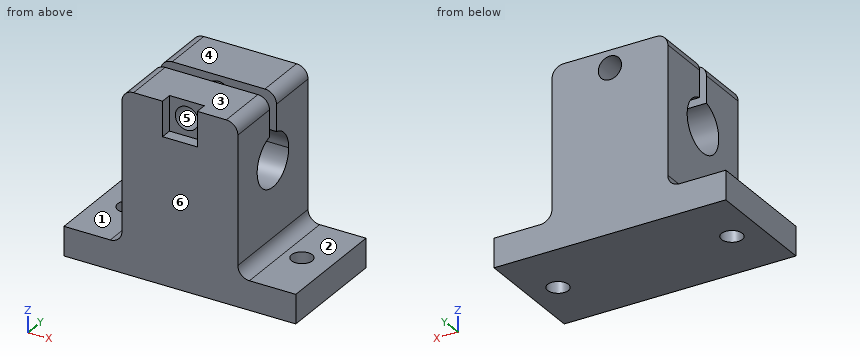
from build123d import *

# Parameters (mm, degrees)
F1_DEPTH = 20
F2_R     = 1.8
F3_DEPTH = 25
F5_DEPTH = 25
F7_DEPTH = 6
F8_R     = 2
F9_DEPTH = 25
F10_R    = 2


with BuildPart() as f1:
    # F0 (on Front) → F1 (new body)
    with BuildSketch(Plane.XZ):
        Polygon((10, 31), (-10, 31), (-10, 5), (-20, 5), (-20, 0), (20, 0), (20, 5), (10, 5), align=None)
    extrude(amount=F1_DEPTH)

    # F2 (on face) → F3 (cut)
    with BuildSketch(Plane(origin=(0, 0, 0), x_dir=(1, 0, 0), z_dir=(0, 0, -1))):
        with Locations((-15, 10)):
            Circle(F2_R)
        with Locations((15, 10)):
            Circle(F2_R)
    extrude(amount=-F3_DEPTH, mode=Mode.SUBTRACT)

    # F4 (on face) → F5 (cut)
    with BuildSketch(Plane.YZ.offset(10)):
        with BuildLine():
            ThreePointArc((-11, 24.3874821937), (-12.8062430401, 16.4821881801), (-5.5, 20))
            ThreePointArc((-5.5, 20), (-6.4821881801, 22.8062430401), (-9, 24.3874821937))
            Line((-9, 24.3874821937), (-9, 20))
            Line((-9, 20), (-10, 20))
            Line((-10, 20), (-11, 20))
            Line((-11, 20), (-11, 24.3874821937))
        make_face()
        with BuildLine():
            ThreePointArc((-11, 24.3874821937), (-10, 24.5), (-9, 24.3874821937))
            Line((-9, 24.3874821937), (-9, 31))
            Line((-9, 31), (-11, 31))
            Line((-11, 31), (-11, 24.3874821937))
        make_face()
        with BuildLine():
            Line((-9, 20), (-9, 24.3874821937))
            ThreePointArc((-9, 24.3874821937), (-10, 24.5), (-11, 24.3874821937))
            Line((-11, 24.3874821937), (-11, 20))
            Line((-11, 20), (-10, 20))
            Line((-10, 20), (-9, 20))
        make_face()
    extrude(amount=-F5_DEPTH, mode=Mode.SUBTRACT)

    # F6 (on face) → F7 (cut)
    with BuildSketch(Plane.XY.offset(31)):
        Polygon((-3, -18), (-3, -20), (3, -20), (3, -18), (0, -18), align=None)
    extrude(amount=-F7_DEPTH, mode=Mode.SUBTRACT)

    # F8 (on face) → F9 (cut)
    with BuildSketch(Plane.XZ.offset(18)):
        with Locations((0, 28)):
            Circle(F8_R)
    extrude(amount=-F9_DEPTH, mode=Mode.SUBTRACT)

    # F10
    f10_edges = [f1.edges().sort_by_distance(p)[0] for p in [
        (10, -15.5, 31),
        (10, -4.5, 31),
        (-10, -4.5, 31),
        (-10, -15.5, 31),
        (10, -10, 5),
        (-10, -10, 5),
    ]]
    fillet(f10_edges, radius=F10_R)


solid = f1.part
Read the model definition and answer for the solid it produces. Units are mm, in the model's axes. Face numbers are marked on the shaded views. A direction names the side the tool comes from. Give positions to 0.01 mm unless a question says otherwise; leave off trailing zeros. Loops run counter-clockwise (first coordinate to the right, second up) from the corner with the lowest first, then second, coordinate; pieces in that order, holes last. Notation, with made-up numbers: M 12,60.25 L 46,60.25 A30 ccw 46,87.25 Z; hole C -25.5,89.5 d10. An arc over 180 degrees is marked long. Write each question's results on one line, items separated by ' | '.
1. Section A-A on y = -10 is taken. Give the vertices of the cut face in (x, z).
Values:
outline: M -20,0 L -16.8,0 L -16.8,5 L -20,5 Z; M -13.2,0 L 13.2,0 L 13.2,5 L 12,5 A2 cw 10,7 L 10,15.5 L -10,15.5 L -10,7 A2 cw -12,5 L -13.2,5 Z; M 16.8,0 L 20,0 L 20,5 L 16.8,5 Z
2. Section B-B on x = 0 is taken. Give the vertices of the cut face in (y, z).
Values:
outline: M -20,0 L 0,0 L 0,26 L -9,26 L -9,24.39 A4.5 cw long -11,24.39 L -11,26 L -18,26 L -18,25 L -20,25 Z; M -18,30 L -11,30 L -11,31 L -18,31 Z; M -9,30 L 0,30 L 0,31 L -9,31 Z
3. Section C-C on y = -15.5 is taken. Give the vertices of the cut face in (x, z), plus the area to 3 significant figures.
Values:
outline: M -20,0 L 20,0 L 20,5 L 12,5 A2 cw 10,7 L 10,29 A2 ccw 8,31 L -8,31 A2 ccw -10,29 L -10,7 A2 cw -12,5 L -20,5 Z; hole C 0,28 d4 | area: 707 mm^2
4. The mould has two halves that part along Z. Classify the marked faces 4, 5 and 6: pulls with the +Z half, pulls with the -Z half, needs draft (parallel to the pull), parting line crosses it, or undercut.
Values:
face 4: pulls with the +Z half | face 5: undercut | face 6: needs draft
5. Straight lines are drawn through the part: line 1 (Y direction, x = -4, z = 20); line 2 (X direction, y = -17, z = 24.5); line 3 (Y direction, x = 4.5, z = 18). For each, find the intervals that lie inside material, in ascending order. Write a range as [from, to].
Values:
line 1: y = [-20, -14.5], [-5.5, 0] | line 2: x = [-10, 10] | line 3: y = [-20, -14.03], [-5.97, 0]
6. Section D-D on x = 15 is taken. Give the vertices of the cut face in (y, z).
Values:
outline: M -20,0 L -11.8,0 L -11.8,5 L -20,5 Z; M -8.2,0 L 0,0 L 0,5 L -8.2,5 Z
7. Given pin 1 (1 mm diameter, centred on x = 1, y = -19.5, fed in from +Z); pin 2 (1.5 mm diameter, centred on y = -5.5, z = 18.5, fed in from -X); pin 3 (11.5 mm diameter, centred on y = -10, z = 20, fed in from +X); pin 4 (3 mm diameter, centred on x = -15, y = -10, fed in from -Z), each flat-ended and moving along its own axis, determine where each tip first touches the part or whether it passes through.
Values:
pin 1: stops at z = 25 | pin 2: stops at x = -10 | pin 3: stops at x = 10 | pin 4: passes through
8. A tool of negligible diameter and unlimited length cuts with its end or side. For the marked faces 1, 2 and 3, from which of +Z, -Z, +X, -X, +Y, -Y can it reach the whole face along a straight path? Write none if from no direction.
Values:
face 1: +Z, -X, +Y, -Y | face 2: +Z, +X, +Y, -Y | face 3: +Z, +X, -X, +Y, -Y
